Verification items for this drawing (mm, ordinates from the low corner). Give positions to 0.01 mm unless a question says otherwise; leave off trailing zeros. Write each loop counter-clockwise with the first axis right and the second up, starting at its lowest first coordinate (ties: lowest second). Pieces come first, ordered by that corner, then holes. Notation, with made-up numbers: (43.5, 55.25) -> (84.5, 55.25) arc R9 ccw to (84.5, 66.25) -> close; hole circle Ø5 at (-33.75, 80.25). An arc over 180 degrees is marked (long way). One line per item, written item: value.
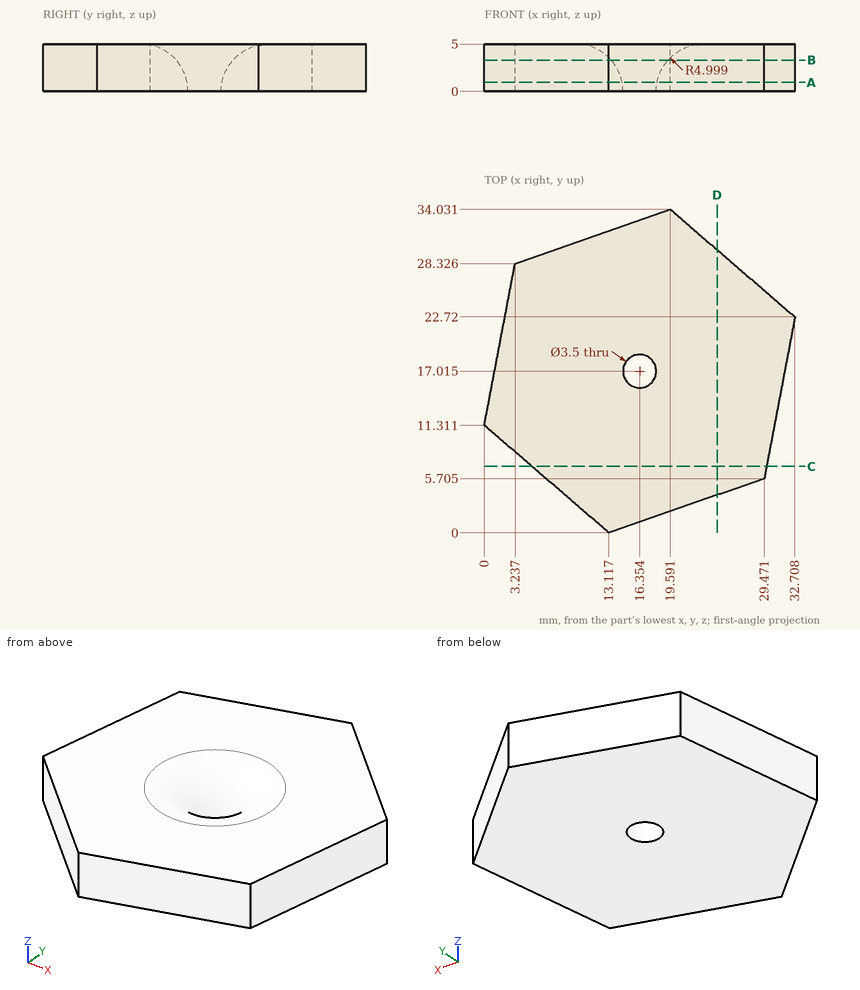
1) Sectioned sample at C-C on y = 7. Record the cut outline in (x, z), plus the area to 3 significant figures.
Verdict:
outline: (5, 0) -> (29.72, 0) -> (29.72, 5) -> (5, 5) -> close
area: 124 mm^2
2) Scan lines: probe 1 along X at (y, z) = (15.5, 2.85) (1 decimal); probe 2 along X at (y, z) = (16, 0.8); probe 3 along Y at (x, z) = (16, 2) (1 decimal). Record each from-to range of solid material in increasing order.
Verdict:
probe 1: 0.8 to 14.2, 18.5 to 31.3
probe 2: 0.89 to 14.85, 17.86 to 31.43
probe 3: 1 to 14.9, 19.2 to 32.8
3) Sectioned sample at B-B on z = 3.3. Record the cut outline in (x, y) (1 decimal), plus the area to 3 significant figures.
Verdict:
outline: (0, 11.3) -> (13.1, 0) -> (29.5, 5.7) -> (32.7, 22.7) -> (19.6, 34) -> (3.2, 28.3) -> close; hole circle Ø6 at (16.4, 17)
area: 751 mm^2
4) Depth check by flat-ended pin: pin 1 Ø2 at (y, z) = (10.5, 3.5) entering from +X; pin 2 Ø12 at (x, y) = (27.5, 5) entering from -Z; pin 3 Ø1 at (y, z) = (3.5, 4.5) entering from -X; pin 4 Ø1 at (x, z) = (22.5, 1.5) entering from -Y. Enter the tip coordinate at first touch or a pass-through.
Verdict:
pin 1: x = 30.57
pin 2: z = 0
pin 3: x = 8.48
pin 4: y = 3.1
5) Sectioned sample at D-D on x = 24.5. Record the cut outline in (y, z), plus the area to 3 significant figures.
Verdict:
outline: (3.97, 0) -> (29.8, 0) -> (29.8, 5) -> (3.97, 5) -> close
area: 129 mm^2
6) Sectioned sample at A-A on z = 0.95. Record the cut outline in (x, y) (1 decimal), plus the area to 3 significant figures.
Verdict:
outline: (0, 11.3) -> (13.1, 0) -> (29.5, 5.7) -> (32.7, 22.7) -> (19.6, 34) -> (3.2, 28.3) -> close; hole circle Ø3.7 at (16.4, 17)
area: 769 mm^2
